from build123d import *

# Parameters (mm, degrees)
F0_W     = 77
F0_H     = 55
F1_DEPTH = 27
F2_W     = 71.92
F2_H     = 49.92
F3_DEPTH = 27
F4_W     = 49.92
F4_H     = 21.92
F5_DEPTH = 127
F6_W     = 71.92
F6_H     = 21.92
F7_DEPTH = 70.104


with BuildPart() as f1:
    # F0 (on Top) → F1 (new body)
    with BuildSketch(Plane.XY):
        with Locations((3.67788, 15.154595)):
            Rectangle(F0_W, F0_H)
    extrude(amount=F1_DEPTH)

    # F2 (on face) → F3 (cut)
    with BuildSketch(Plane.XY.offset(27)):
        with Locations((3.67788, 15.154595)):
            Rectangle(F2_W, F2_H)
    extrude(amount=-F3_DEPTH, mode=Mode.SUBTRACT)

    # F4 (on face) → F5 (cut)
    with BuildSketch(Plane.YZ.offset(42.17788)):
        with Locations((15.154595, 13.5)):
            Rectangle(F4_W, F4_H)
    extrude(amount=-F5_DEPTH, mode=Mode.SUBTRACT)

    # F6 (on face) → F7 (cut)
    with BuildSketch(Plane.XZ.offset(12.345405)):
        with Locations((3.67788, 13.5)):
            Rectangle(F6_W, F6_H)
    extrude(amount=-F7_DEPTH, mode=Mode.SUBTRACT)


solid = f1.part
Can you work these out from the model? Positions are in its coordinate system, mm. A direction names the side the tool comes from. Round coordinates to 2 decimals unless told otherwise and drop trailing zeros. Write each loop counter-clockwise with the first axis right and the second up, starting at its lowest first coordinate (ties: lowest second). Pieces come first, ordered by that corner, then holes. Notation, with made-up numbers: M 5.5,19 L 18.5,19 A27 cw 18.5,43 Z; hole C -12,44.5 d1. An arc over 180 degrees is marked long. Use CSV: the item, a comma, the result in double quotes.
(1) I need wall thicknesses on line 1 along Y through (x, z) = (24, 24.5). Which ranges of the line are inside material? Lowest first, please.
Check values:
line 1,"-12.35 to -9.81, 40.11 to 42.65"
(2) We'd pull the mould along Y, two halves only. Please class faces 1 (the flat face through (6, 42.655, 2)), 2 (the flat face through (4, -9.805, 26)), 3 (the flat face through (41, -9.805, 13)), 4 (the flat face through (1, -11, 27)): +Y half, -Y half, draft (parallel to the pull), parting line (faces both ways), or undercut.
Check values:
face 1,"+Y half"
face 2,"undercut"
face 3,"undercut"
face 4,"draft"
(3) Imagine slicing it at A-A (y = 4). Write out the boundary of the cut face in (x, z).
Check values:
outline,"M -34.82,0 L -32.28,0 L -32.28,2.54 L -34.82,2.54 Z; M -34.82,24.46 L -32.28,24.46 L -32.28,27 L -34.82,27 Z; M 39.64,0 L 42.18,0 L 42.18,2.54 L 39.64,2.54 Z; M 39.64,24.46 L 42.18,24.46 L 42.18,27 L 39.64,27 Z"
(4) Imagine slicing it at B-B (x = 27). Write out the boundary of the cut face in (y, z).
Check values:
outline,"M -12.35,0 L -9.81,0 L -9.81,2.54 L -12.35,2.54 Z; M -12.35,24.46 L -9.81,24.46 L -9.81,27 L -12.35,27 Z; M 40.11,0 L 42.65,0 L 42.65,2.54 L 40.11,2.54 Z; M 40.11,24.46 L 42.65,24.46 L 42.65,27 L 40.11,27 Z"
(5) On a 3-axis mill with a long thin cutter (end or side, diameter ignored), from which of +Z, -Z, +X, -X, +Y, -Y can I reach the whole of each face in a straight line? I mean faces 5 (the flat face through (-34, 15, 24.46)), 6 (the flat face through (3, -11, 2.54)), 7 (the flat face through (-32.282, 15, 1)). Say none if no direction works.
Check values:
face 5,"+X, -X"
face 6,"+Y, -Y"
face 7,"+Z, -Z"
